```python
from build123d import *

# Parameters (mm, degrees)
SKETCH_1_R          = 17.5
EXTRUDE_1_DEPTH     = 27.3
SKETCH_2_R          = 4.85
EXTRUDE_2_DEPTH     = 2.5
SKETCH_3_R          = 2.5
EXTRUDE_3_DEPTH     = 4.6
EXTRUDE_4_DEPTH     = 9
EXTRUDE_5_DEPTH     = 23.4
SKETCH_6_R          = 2.1
EXTRUDE_6_DEPTH     = 1.05
CUT_EXTRUDE_1_DEPTH = 1.05
SKETCH_8_R          = 0.5
EXTRUDE_7_DEPTH     = 10


with BuildPart() as part:
    # 草图1 → 凸台-拉伸1 (new body)
    with BuildSketch(Plane.XY):
        Circle(SKETCH_1_R)
    extrude(amount=EXTRUDE_1_DEPTH)

    # 草图2 → 凸台-拉伸2 (add)
    with BuildSketch(Plane(origin=(0, 0, 0), x_dir=(-1, 0, 0), z_dir=(0, 0, -1))):
        Circle(SKETCH_2_R)
    extrude(amount=EXTRUDE_2_DEPTH)

    # 草图3 → 凸台-拉伸3 (add)
    with BuildSketch(Plane(origin=(0, 0, -2.5), x_dir=(-1, 0, 0), z_dir=(0, 0, -1))):
        Circle(SKETCH_3_R)
    extrude(amount=EXTRUDE_3_DEPTH)

    # 草图4 → 凸台-拉伸4 (add)
    with BuildSketch(Plane(origin=(0, 0, -7.1), x_dir=(-1, 0, 0), z_dir=(0, 0, -1))):
        with BuildLine():
            Line((2.022152319, 1.47), (-2.022152319, 1.47))
            ThreePointArc((-2.022152319, 1.47), (-2.5, 0), (-2.022152319, -1.47))
            Line((-2.022152319, -1.47), (2.022152319, -1.47))
            ThreePointArc((2.022152319, -1.47), (2.377538727, -0.772858073), (2.5, 0))
            ThreePointArc((2.5, 0), (2.377538727, 0.772858073), (2.022152319, 1.47))
        make_face()
    extrude(amount=EXTRUDE_4_DEPTH)

    # 草图5 → 凸台-拉伸5 (add)
    with BuildSketch(Plane(origin=(0, 0, 0), x_dir=(-1, 0, 0), z_dir=(0, 0, -1))):
        with BuildLine():
            ThreePointArc((8.8, -15.126466871), (0, -17.5), (-8.8, -15.126466871))
            Line((-8.8, -15.126466871), (-8.8, -23.08))
            Line((-8.8, -23.08), (8.8, -23.08))
            Line((8.8, -23.08), (8.8, -15.126466871))
        make_face()
    extrude(amount=-EXTRUDE_5_DEPTH)

    # 草图6 → 凸台-拉伸6 (add)
    # profile 1 of 6: a face of its own
    with BuildSketch(Plane(origin=(0, 0, 0), x_dir=(-1, 0, 0), z_dir=(0, 0, -1))):
        with BuildLine():
            ThreePointArc((-13.433971222, -11.215097736), (-15.650847937, -11.032512316), (-17.606958852, -12.091525958))
            ThreePointArc((-17.606958852, -12.091525958), (-17.606958852, -17.606958852), (-12.091525958, -17.606958852))
            ThreePointArc((-12.091525958, -17.606958852), (-11.246112228, -16.341707791), (-10.949242405, -14.849242405))
            ThreePointArc((-10.949242405, -14.849242405), (-11.016282438, -14.129229978), (-11.215097736, -13.433971222))
            ThreePointArc((-11.215097736, -13.433971222), (-12.374368671, -12.374368671), (-13.433971222, -11.215097736))
        make_face()
        with Locations((-14.849242405, -14.849242405)):
            Circle(SKETCH_6_R, mode=Mode.SUBTRACT)
    # profile 2 of 6: a face of its own
    with BuildSketch(Plane(origin=(0, 0, 0), x_dir=(-1, 0, 0), z_dir=(0, 0, -1))):
        with BuildLine():
            ThreePointArc((-10.949242405, -14.849242405), (-11.246112228, -16.341707791), (-12.091525958, -17.606958852))
            Line((-12.091525958, -17.606958852), (-9.305450633, -14.820883527))
            ThreePointArc((-9.305450633, -14.820883527), (-10.283681626, -14.159657207), (-11.215097736, -13.433971222))
            ThreePointArc((-11.215097736, -13.433971222), (-11.016282438, -14.129229978), (-10.949242405, -14.849242405))
        make_face()
    # profile 3 of 6: a face of its own
    with BuildSketch(Plane(origin=(0, 0, 0), x_dir=(-1, 0, 0), z_dir=(0, 0, -1))):
        with BuildLine():
            ThreePointArc((-13.433971222, -11.215097736), (-14.159657207, -10.283681626), (-14.820883527, -9.305450633))
            Line((-14.820883527, -9.305450633), (-17.606958852, -12.091525958))
            ThreePointArc((-17.606958852, -12.091525958), (-15.650847937, -11.032512316), (-13.433971222, -11.215097736))
        make_face()
    # profile 4 of 6: a face of its own
    with BuildSketch(Plane(origin=(0, 0, 0), x_dir=(-1, 0, 0), z_dir=(0, 0, -1))):
        with BuildLine():
            ThreePointArc((18.749242405, 14.849242405), (16.341707791, 18.452372582), (12.091525958, 17.606958852))
            ThreePointArc((12.091525958, 17.606958852), (11.032512316, 15.650847937), (11.215097736, 13.433971222))
            ThreePointArc((11.215097736, 13.433971222), (12.374368671, 12.374368671), (13.433971222, 11.215097736))
            ThreePointArc((13.433971222, 11.215097736), (15.650847937, 11.032512316), (17.606958852, 12.091525958))
            ThreePointArc((17.606958852, 12.091525958), (18.452372582, 13.356777019), (18.749242405, 14.849242405))
        make_face()
        with Locations((14.849242405, 14.849242405)):
            Circle(SKETCH_6_R, mode=Mode.SUBTRACT)
    # profile 5 of 6: a face of its own
    with BuildSketch(Plane(origin=(0, 0, 0), x_dir=(-1, 0, 0), z_dir=(0, 0, -1))):
        with BuildLine():
            ThreePointArc((17.606958852, 12.091525958), (15.650847937, 11.032512316), (13.433971222, 11.215097736))
            ThreePointArc((13.433971222, 11.215097736), (14.159657207, 10.283681626), (14.820883527, 9.305450633))
            Line((14.820883527, 9.305450633), (17.606958852, 12.091525958))
        make_face()
    # profile 6 of 6: a face of its own
    with BuildSketch(Plane(origin=(0, 0, 0), x_dir=(-1, 0, 0), z_dir=(0, 0, -1))):
        with BuildLine():
            Line((12.091525958, 17.606958852), (9.305450633, 14.820883527))
            ThreePointArc((9.305450633, 14.820883527), (10.283681626, 14.159657207), (11.215097736, 13.433971222))
            ThreePointArc((11.215097736, 13.433971222), (11.032512316, 15.650847937), (12.091525958, 17.606958852))
        make_face()
    extrude(amount=-EXTRUDE_6_DEPTH)

    # 草图7 → 切除-拉伸1 (cut)
    with BuildSketch(Plane.XZ.offset(23.08)):
        with BuildLine():
            Line((-2, 6.6), (2, 6.6))
            ThreePointArc((2, 6.6), (2.8, 5.8), (2, 5))
            Line((2, 5), (-2, 5))
            ThreePointArc((-2, 5), (-2.8, 5.8), (-2, 6.6))
        make_face()
    extrude(amount=-CUT_EXTRUDE_1_DEPTH, mode=Mode.SUBTRACT)

    # 草图8 → 凸台-拉伸7 (add)
    with BuildSketch(Plane.XZ.offset(22.03)):
        with Locations(Location((2.287967864, 5.8, 0), (0, 0, 270))):
            Circle(SKETCH_8_R)
        with Locations(Location((1.167967864, 5.8, 0), (0, 0, 270))):
            Circle(SKETCH_8_R)
        with Locations(Location((0.047967864, 5.8, 0), (0, 0, 270))):
            Circle(SKETCH_8_R)
        with Locations(Location((-1.072032136, 5.8, 0), (0, 0, 270))):
            Circle(SKETCH_8_R)
        with Locations(Location((-2.192032136, 5.8, 0), (0, 0, 270))):
            Circle(SKETCH_8_R)
    extrude(amount=EXTRUDE_7_DEPTH)


solid = part.part
```
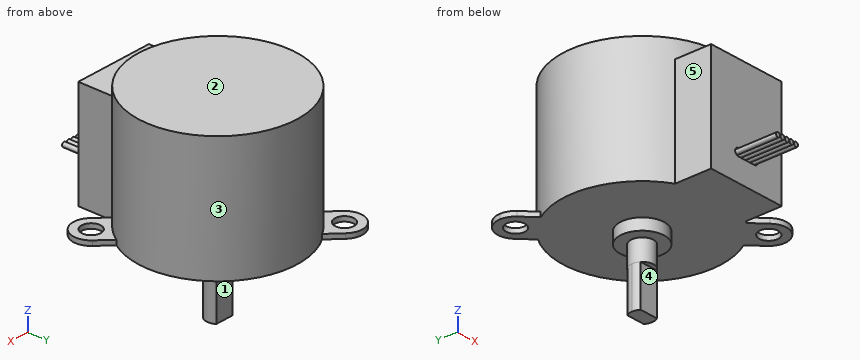
Part model, mm, in its own coordinate system. Face numbers are marked on the shaded views. A direction names the side the tool comes from. Round coordinates to 2 decimals unless told otherwise and drop trailing zeros. Loops run counter-clockwise (first coordinate to the right, second up) from the corner with the lowest first, then second, coordinate; pieces in that order, holes last.
Item 1: Drop flat-ended pins along their axis: P1, Ø10, axis at y = -17.5, z = 0.5, coming from the -X side; P2, Ø2.5, axis at y = -17.5, z = 14.5, coming from the +X side; P3, Ø6, axis at y = -15, z = 2, coming from the -X side; P4, Ø5, axis at x = 2.5, y = -1, coming from the -Z side. Give the stop position or say it passes through.
Item 2: Cut at A-A, the plane z = -10.5. Give the cut face in (x, y), then the cut area to 3 significant figures.
Item 3: Cut at B-B, the plane z = -4. Give the cut face in (x, y).
Item 4: Drill centre lines: line 1 (Z direction, x = 9.5, y = 13.5); line 2 (X direction, y = -18, z = 15); line 3 (Y direction, x = -12, z = 24). Where is each one in solid material? Low to high.
Item 5: Cut at C-C, the plane z = 11. Give the cut face in (x, y), then the cut area to 3 significant figures.
Item 6: 3-axis set-ups, long thin cutter, end or side, ignore diameter. For the marked faces 1, 2, 3, 4 and 5: which of +Z, -Z, +X, -X, +Y, -Y reach the whole face in a straight line?
A:
1. P1: stops at x = -12.25
1. P2: stops at x = 8.8
1. P3: stops at x = -12.74
1. P4: stops at z = -16.1
2. outline: (-2.02, -1.47) - (2.02, -1.47) arc R2.5 ccw to (2.02, 1.47) - (-2.02, 1.47) arc R2.5 ccw to start
2. area: 13.8 mm2
3. outline: circle Ø5 at (0, 0)
4. line 1: z = 0 to 27.3
4. line 2: x = -8.8 to 8.8
4. line 3: y = -12.74 to 12.74
5. outline: (-8.8, -23.08) - (8.8, -23.08) - (8.8, -15.13) arc R17.5 ccw (long way) to (-8.8, -15.13) - close
5. area: 1,070 mm2
6. face 1: -Z, +X, -X, +Y
6. face 2: +Z, +X, -X, +Y, -Y
6. face 3: +Z
6. face 4: -Z, +X, -X, -Y
6. face 5: +Z, -Z, -X, -Y
